```python
from build123d import *

# Parameters (mm, degrees)
SKETCH_1_W           = 30
SKETCH_1_H           = 11
EXTRUDE_1_DEPTH      = 6
SKETCH_2_W           = 16
SKETCH_2_H           = 2
CUT_EXTRUDE_1_DEPTH  = 144
EXTRUDE_2_DEPTH      = 50
SKETCH_4_R           = 1.75
CUT_EXTRUDE_2_DEPTH  = 144
SKETCH_5_W           = 11
SKETCH_5_H           = 56
CUT_EXTRUDE_3_DEPTH  = 2.5
SKETCH_7_W           = 11
SKETCH_7_H           = 54
CUT_EXTRUDE_5_DEPTH  = 47
EXTRUDE_3_DEPTH      = 16
EXTRUDE_3_DEPTH_BACK = 2
SKETCH_8_W           = 27.5
SKETCH_8_H           = 1.482402205
SKETCH_9_W           = 27.5
SKETCH_9_H           = 3
EXTRUDE_4_DEPTH      = 16
SKETCH_10_W          = 3
SKETCH_10_H          = 18
CUT_EXTRUDE_6_DEPTH  = 47
SKETCH_12_W          = 27.5
SKETCH_12_H          = 3
EXTRUDE_5_DEPTH      = 15.5
SKETCH_13_W          = 27.5
SKETCH_13_H          = 2
EXTRUDE_6_DEPTH      = 53
SKETCH_14_W          = 27.5
SKETCH_14_H          = 18.982402205
EXTRUDE_7_DEPTH      = 3
SKETCH_15_W          = 27.5
SKETCH_15_H          = 2
EXTRUDE_8_DEPTH      = 13
SKETCH_16_W          = 27.5
SKETCH_16_H          = 10
EXTRUDE_9_DEPTH      = 2
CUT_EXTRUDE_START    = -6
SKETCH_17_R          = 1.75
CUT_EXTRUDE_8_DEPTH  = 6
FILLET_1_R           = 10
FILLET_2_R           = 2
CUT_EXTRUDE_9_DEPTH  = 63
SKETCH_19_W          = 18.982402205
SKETCH_19_H          = 16.821441914
CUT_EXTRUDE_10_DEPTH = 63


with BuildPart() as part:
    # 草图1 → 凸台-拉伸1 (new body)
    with BuildSketch(Plane(origin=(0, 0, 0), x_dir=(1, 0, 0), z_dir=(0, 1, 0))):
        Rectangle(SKETCH_1_W, SKETCH_1_H)
    extrude(amount=EXTRUDE_1_DEPTH)

    # 草图2 → 切除-拉伸1 (cut)
    with BuildSketch(Plane.ZY.offset(15)):
        with Locations((-5.5, 3)):
            Rectangle(SKETCH_2_W, SKETCH_2_H)
    extrude(amount=-CUT_EXTRUDE_1_DEPTH, mode=Mode.SUBTRACT)

    # 草图3 → 凸台-拉伸2 (add)
    with BuildSketch(Plane(origin=(0, 6, 0), x_dir=(1, 0, 0), z_dir=(0, 1, 0))):
        Polygon((2, 5.5), (-2, 5.5), (-2, -3.5), (-15, -3.5), (-15, -5.5), (15, -5.5), (15, -3.5), (2, -3.5), align=None)
    extrude(amount=EXTRUDE_2_DEPTH)

    # 草图4 → 切除-拉伸2 (cut)
    with BuildSketch(Plane(origin=(0, 6, 0), x_dir=(1, 0, 0), z_dir=(0, 1, 0))):
        with Locations(Location((-7.5, 2, 0), (0, 0, 270))):
            Circle(SKETCH_4_R)
        with Locations(Location((7.5, 2, 0), (0, 0, 270))):
            Circle(SKETCH_4_R)
    extrude(amount=-CUT_EXTRUDE_2_DEPTH, mode=Mode.SUBTRACT)

    # 草图5 → 切除-拉伸3 (cut)
    with BuildSketch(Plane.ZY.offset(15)):
        with Locations((0, 28)):
            Rectangle(SKETCH_5_W, SKETCH_5_H)
    extrude(amount=-CUT_EXTRUDE_3_DEPTH, mode=Mode.SUBTRACT)

    # 草图7 → 切除-拉伸5 (cut)
    with BuildSketch(Plane.ZY.offset(12.5)):
        with Locations((0, 29)):
            Rectangle(SKETCH_7_W, SKETCH_7_H)
    extrude(amount=-CUT_EXTRUDE_5_DEPTH, mode=Mode.SUBTRACT)

    # 草图8 → 凸台-拉伸3 (add, two sides: drawn at the far end of the back side and taken through both)
    with BuildSketch(Plane(origin=(0, 2, 0), x_dir=(1, 0, 0), z_dir=(0, 1, 0)).offset(-EXTRUDE_3_DEPTH_BACK)):
        with Locations((1.25, -6.241201102)):
            Rectangle(SKETCH_8_W, SKETCH_8_H)
    extrude(amount=EXTRUDE_3_DEPTH + EXTRUDE_3_DEPTH_BACK)

    # 草图9 → 凸台-拉伸4 (add)
    with BuildSketch(Plane(origin=(0, 2, 0), x_dir=(1, 0, 0), z_dir=(0, 1, 0))):
        with Locations((1.25, -4)):
            Rectangle(SKETCH_9_W, SKETCH_9_H)
    extrude(amount=EXTRUDE_4_DEPTH)

    # 草图10 → 切除-拉伸6 (cut)
    with BuildSketch(Plane(origin=(15, 0, 0), x_dir=(0, 0, -1), z_dir=(1, 0, 0))):
        with Locations((-5.482402205, 9)):
            Rectangle(SKETCH_10_W, SKETCH_10_H)
    extrude(amount=-CUT_EXTRUDE_6_DEPTH, mode=Mode.SUBTRACT)

    # 草图12 → 凸台-拉伸5 (add)
    with BuildSketch(Plane.XY.offset(3.982402205)):
        with Locations((1.25, 16.5)):
            Rectangle(SKETCH_12_W, SKETCH_12_H)
    extrude(amount=EXTRUDE_5_DEPTH)

    # 草图13 → 凸台-拉伸6 (add)
    with BuildSketch(Plane(origin=(0, 15, 0), x_dir=(-1, 0, 0), z_dir=(0, -1, 0))):
        with Locations((-1.25, -20.482402205)):
            Rectangle(SKETCH_13_W, SKETCH_13_H)
    extrude(amount=-EXTRUDE_6_DEPTH)

    # 草图14 → 凸台-拉伸7 (add)
    with BuildSketch(Plane(origin=(0, 68, 0), x_dir=(1, 0, 0), z_dir=(0, 1, 0))):
        with Locations((1.25, -11.991201102)):
            Rectangle(SKETCH_14_W, SKETCH_14_H)
    extrude(amount=EXTRUDE_7_DEPTH)

    # 草图15 → 凸台-拉伸8 (add)
    with BuildSketch(Plane(origin=(0, 71, 0), x_dir=(1, 0, 0), z_dir=(0, 1, 0))):
        with Locations((1.25, -3.5)):
            Rectangle(SKETCH_15_W, SKETCH_15_H)
    extrude(amount=EXTRUDE_8_DEPTH)

    # 草图16 → 凸台-拉伸9 (add)
    with BuildSketch(Plane(origin=(0, 84, 0), x_dir=(1, 0, 0), z_dir=(0, 1, 0))):
        with Locations((1.25, 0.5)):
            Rectangle(SKETCH_16_W, SKETCH_16_H)
    extrude(amount=EXTRUDE_9_DEPTH)

    # 草图17 → 切除-拉伸8 (cut)
    with BuildSketch(Plane(origin=(0, 84, 0), x_dir=(-1, 0, 0), z_dir=(0, -1, 0)).offset(CUT_EXTRUDE_START)):
        with Locations(Location((7.5, 2, 0), (0, 0, 270))):
            Circle(SKETCH_17_R)
        with Locations(Location((-7.5, 2, 0), (0, 0, 270))):
            Circle(SKETCH_17_R)
    extrude(amount=CUT_EXTRUDE_8_DEPTH, mode=Mode.SUBTRACT)

    # 圆角1
    fillet_1_edges = [part.edges().sort_by_distance(p)[0] for p in [
        (1.25, 15, 3.982402205),
        (1.25, 71, 4.5),
    ]]
    fillet(fillet_1_edges, radius=FILLET_1_R)

    # 圆角2
    # the kernel refuses this fillet: 2 mm, written as the material it takes off along each edge
    with BuildSketch(Plane(origin=(-12.5, -5, 3.982402205), x_dir=(1, 0, 0), z_dir=(0, 1, 0)), Plane(origin=(-12.5, 81, 4.5), x_dir=(1, 0, 0), z_dir=(0, 1, 0))) as fillet_2_piece_1:
        with BuildLine():
            CenterArc((FILLET_2_R, FILLET_2_R), FILLET_2_R, 180, 90)
            Line((0, FILLET_2_R), (0, 0))
            Line((0, 0), (FILLET_2_R, 0))
        make_face()
    extrude(amount=10, mode=Mode.SUBTRACT)
    with BuildSketch(Plane(origin=(15, 5, 3.982402205), x_dir=(0, 0, -1), z_dir=(0, -1, 0)), Plane(origin=(15, 91, 4.5), x_dir=(0, 0, -1), z_dir=(0, -1, 0))) as fillet_2_piece_2:
        with BuildLine():
            CenterArc((FILLET_2_R, -FILLET_2_R), FILLET_2_R, 90, 90)
            Line((0, -FILLET_2_R), (0, 0))
            Line((0, 0), (FILLET_2_R, 0))
        make_face()
    extrude(amount=10, mode=Mode.SUBTRACT)
    with BuildSketch(Plane(origin=(-12.5, 15, 13.982402205), x_dir=(1, 0, 0), z_dir=(0, 0, 1))) as fillet_2_piece_3:
        with BuildLine():
            CenterArc((FILLET_2_R, FILLET_2_R), FILLET_2_R, 180, 90)
            Line((0, FILLET_2_R), (0, 0))
            Line((0, 0), (FILLET_2_R, 0))
        make_face()
    extrude(amount=12.5, mode=Mode.SUBTRACT)
    with BuildSketch(Plane(origin=(15, 15, 26.482402205), x_dir=(0, 1, 0), z_dir=(0, 0, -1))) as fillet_2_piece_4:
        with BuildLine():
            CenterArc((FILLET_2_R, -FILLET_2_R), FILLET_2_R, 90, 90)
            Line((0, -FILLET_2_R), (0, 0))
            Line((0, 0), (FILLET_2_R, 0))
        make_face()
    extrude(amount=12.5, mode=Mode.SUBTRACT)
    with BuildSketch(Plane(origin=(20, 15, 21.482402205), x_dir=(0, 1, 0), z_dir=(-1, 0, 0))) as fillet_2_piece_5:
        with BuildLine():
            CenterArc((FILLET_2_R, FILLET_2_R), FILLET_2_R, 180, 90)
            Line((0, FILLET_2_R), (0, 0))
            Line((0, 0), (FILLET_2_R, 0))
        make_face()
    extrude(amount=37.5, mode=Mode.SUBTRACT)
    with BuildSketch(Plane(origin=(-17.5, 71, 21.482402205), x_dir=(0, 0, -1), z_dir=(1, 0, 0))) as fillet_2_piece_6:
        with BuildLine():
            CenterArc((FILLET_2_R, -FILLET_2_R), FILLET_2_R, 90, 90)
            Line((0, -FILLET_2_R), (0, 0))
            Line((0, 0), (FILLET_2_R, 0))
        make_face()
    extrude(amount=37.5, mode=Mode.SUBTRACT)
    with BuildSketch(Plane(origin=(15, 71, 26.482402205), x_dir=(0, -1, 0), z_dir=(0, 0, -1))) as fillet_2_piece_7:
        with BuildLine():
            CenterArc((FILLET_2_R, FILLET_2_R), FILLET_2_R, 180, 90)
            Line((0, FILLET_2_R), (0, 0))
            Line((0, 0), (FILLET_2_R, 0))
        make_face()
    extrude(amount=11.982402205, mode=Mode.SUBTRACT)
    with BuildSketch(Plane(origin=(-12.5, 71, 14.5), x_dir=(1, 0, 0), z_dir=(0, 0, 1))) as fillet_2_piece_8:
        with BuildLine():
            CenterArc((FILLET_2_R, -FILLET_2_R), FILLET_2_R, 90, 90)
            Line((0, -FILLET_2_R), (0, 0))
            Line((0, 0), (FILLET_2_R, 0))
        make_face()
    extrude(amount=11.982402205, mode=Mode.SUBTRACT)
    with BuildSketch(Plane(origin=(15, 81, 14.5), x_dir=(0, 0, -1), z_dir=(0, 1, 0))) as fillet_2_piece_9:
        with BuildLine():
            CenterArc((10 + FILLET_2_R, FILLET_2_R), FILLET_2_R, 180, 90)
            Line((10, FILLET_2_R), (10, 0))
            Line((10, 0), (10 + FILLET_2_R, 0))
        make_face()
    revolve(axis=Axis((15, 81, 14.5), (-1, 0, 0)), revolution_arc=90, mode=Mode.SUBTRACT)
    with BuildSketch(Plane(origin=(-12.5, 81, 14.5), x_dir=(0, 0, -1), z_dir=(0, 1, 0))) as fillet_2_piece_10:
        with BuildLine():
            CenterArc((10 + FILLET_2_R, -FILLET_2_R), FILLET_2_R, 90, 90)
            Line((10 + FILLET_2_R, 0), (10, 0))
            Line((10, 0), (10, -FILLET_2_R))
        make_face()
    revolve(axis=Axis((-12.5, 81, 14.5), (-1, 0, 0)), revolution_arc=90, mode=Mode.SUBTRACT)
    with BuildSketch(Plane(origin=(15, 5, 13.982402205), x_dir=(0, 0, -1), z_dir=(0, -1, 0))) as fillet_2_piece_11:
        with BuildLine():
            CenterArc((10 + FILLET_2_R, -FILLET_2_R), FILLET_2_R, 90, 90)
            Line((10, -FILLET_2_R), (10, 0))
            Line((10, 0), (10 + FILLET_2_R, 0))
        make_face()
    revolve(axis=Axis((15, 5, 13.982402205), (1, 0, 0)), revolution_arc=90, mode=Mode.SUBTRACT)
    with BuildSketch(Plane(origin=(-12.5, 5, 13.982402205), x_dir=(0, 0, -1), z_dir=(0, -1, 0))) as fillet_2_piece_12:
        with BuildLine():
            CenterArc((10 + FILLET_2_R, FILLET_2_R), FILLET_2_R, 180, 90)
            Line((10 + FILLET_2_R, 0), (10, 0))
            Line((10, 0), (10, FILLET_2_R))
        make_face()
    revolve(axis=Axis((-12.5, 5, 13.982402205), (1, 0, 0)), revolution_arc=90, mode=Mode.SUBTRACT)

    # 草图18 → 切除-拉伸9 (cut)
    with BuildSketch(Plane(origin=(15, 0, 0), x_dir=(0, 0, -1), z_dir=(1, 0, 0))):
        with BuildLine():
            Line((-2.5, 81), (-2.5, 68))
            Line((-2.5, 68), (12.398606428, 68))
            Line((12.398606428, 68), (12.398606428, 90.674751071))
            Line((12.398606428, 90.674751071), (-21.482402205, 90.674751071))
            Line((-21.482402205, 90.674751071), (-21.482402205, 69))
            Line((-21.482402205, 69), (-14.5, 69))
            ThreePointArc((-14.5, 69), (-6.014718626, 72.514718626), (-2.5, 81))
        make_face()
    extrude(amount=-CUT_EXTRUDE_9_DEPTH, mode=Mode.SUBTRACT)

    # 草图19 → 切除-拉伸10 (cut)
    with BuildSketch(Plane(origin=(15, 0, 0), x_dir=(0, 0, -1), z_dir=(1, 0, 0))):
        with Locations((-11.991201102, 76.410720957)):
            Rectangle(SKETCH_19_W, SKETCH_19_H)
    extrude(amount=-CUT_EXTRUDE_10_DEPTH, mode=Mode.SUBTRACT)


solid = part.part
```
The listing builds one solid part. Answer for the finished solid, in the listing's coordinates (mm). A direction names the side the tool comes from. Round coordinates to 2 decimals unless told otherwise and drop trailing zeros. Loops run counter-clockwise (first coordinate to the right, second up) from the corner with the lowest first, then second, coordinate; pieces in that order, holes last.
Q1. Which of the six approach directions +Z, -Z, +X, -X, +Y, -Y give full straight-line access (tool end or side, diameter ignored) to faces 4 (the face through (1, 2, 3.982)), 5 (the face through (1, 2, -2)), 6 (the face through (-11.665, 2.465, 3.608))?
Q2. For a pull along X with two mould halves and no side action, classify faces 1 (the face through (15, 1, -2)), 2 (the face through (1, 1, -5.5)), 3 (the face through (6.83, 1.014, -0.383)) as released by +X, released by -X, zero draft, split by the parting line, or undercut.
Q3. Find the intervals of material crossed by line 1 (X direction, y = 0.9, z = -2); line 2 (Y direction, x = 8, z = 19.25); line 3 (Z direction, x = 12.25, y = 28), in increasing order.
Q4. Section B-B, the plane x = -7.5 is taken. Determine the outline of the cut face in (y, z), then the cut area to 3 significant figures.
Q5. Section C-C, the plane z = 18.75 is taken. Determine the outline of the cut face in (x, y).
Q6. Given pin 1 Ø12 at (x, y) = (7, 34) entering from -Z; pin 2 Ø3 at (x, z) = (1.5, 17) entering from +Y; pin 3 Ø5.5 at (x, y) = (-2, 1.5) entering from +Z, each flat-ended and moving along its own axis, determine where each tip first touches the part or whether it passes through.
Q7. Section A-A, the plane z = -2 is taken. Determine the outline of the cut face in (x, y).
Q8. Section D-D, the plane y = 41.5 is taken. Determine the outline of the cut face in (x, z).
Completed:
1. face 4: +Z, +X, -X, -Y
1. face 5: -Z, +X, -X, +Y
1. face 6: +Z, -X, -Y
2. face 1: released by +X
2. face 2: zero draft
2. face 3: undercut
3. line 1: x = -12.5 to -9.25, -5.75 to 5.75, 9.25 to 15
3. line 2: y = 15 to 18
3. line 3: z = 19.48 to 21.48
4. outline: (0, -5.5) - (2, -5.5) - (2, -3.75) - (0, -3.75) - close; (0, -0.25) - (2, -0.25) - (2, 2.5) - (18, 2.5) - (18, 19.48) - (68, 19.48) - (68, 21.48) - (17, 21.48) arc R2 ccw to (15, 19.48) - (15, 13.98) arc R10 cw to (5, 3.98) - (0, 3.98) - close
4. area: 209 mm2
5. outline: (-12.5, 17) arc R2 ccw to (-10.5, 15) - (13, 15) arc R2 ccw to (15, 17) - (15, 18) - (-12.5, 18) - close
6. pin 1: stops at z = 19.48
6. pin 2: stops at y = 18
6. pin 3: stops at z = 3.98
7. outline: (-12.5, 0) - (-9.25, 0) - (-9.25, 2) - (-12.5, 2) - close; (-5.75, 0) - (5.75, 0) - (5.75, 2) - (-5.75, 2) - close; (9.25, 0) - (15, 0) - (15, 2) - (9.25, 2) - close
8. outline: (-12.5, 19.48) - (15, 19.48) - (15, 21.48) - (-12.5, 21.48) - close
